```python
from build123d import *

# Parameters (mm, degrees)
SKETCH1_W           = 21
SKETCH1_H           = 15
BOSS_EXTRUDE1_DEPTH = 15
SKETCH3_W           = 18
SKETCH3_H           = 7
CUT_EXTRUDE1_DEPTH  = 3
SKETCH4_W           = 7
SKETCH4_H           = 7
BOSS_EXTRUDE3_DEPTH = 9
FILLET2_R           = 1


with BuildPart() as part:
    # Sketch1 → Boss-Extrude1 (new body)
    with BuildSketch(Plane(origin=(0, 0, 0), x_dir=(1, 0, 0), z_dir=(0, 1, 0))):
        Rectangle(SKETCH1_W, SKETCH1_H)
    extrude(amount=BOSS_EXTRUDE1_DEPTH)

    # Sketch3 → Cut-Extrude1 (cut)
    with BuildSketch(Plane(origin=(0, 15, 0), x_dir=(1, 0, 0), z_dir=(0, 1, 0))):
        Rectangle(SKETCH3_W, SKETCH3_H)
    extrude(amount=-CUT_EXTRUDE1_DEPTH, mode=Mode.SUBTRACT)

    # Sketch4 → Boss-Extrude3 (add)
    with BuildSketch(Plane(origin=(0, 12, 0), x_dir=(1, 0, 0), z_dir=(0, 1, 0))):
        with Locations((-5.5, 0)):
            Rectangle(SKETCH4_W, SKETCH4_H)
    extrude(amount=BOSS_EXTRUDE3_DEPTH)

    # Fillet2
    fillet2_edges = [part.edges().sort_by_distance(p)[0] for p in [
        (-9, 21, 0),
        (-5.5, 21, 3.5),
        (-2, 21, 0),
        (-5.5, 21, -3.5),
    ]]
    fillet(fillet2_edges, radius=FILLET2_R)


solid = part.part
```
Check sheet for the modelled part. Datum: model origin and axes. Units: mm. A direction names the side the tool comes from. Coordinates: 2 decimals unless noted, no trailing zeros. Loops run counter-clockwise (first coordinate to the right, second up) from the corner with the lowest first, then second, coordinate; pieces in that order, holes last.
1) Sectioned sample at C-C (y = 13.5). Record the boundary of the cut face in (x, z).
2) Sectioned sample at B-B (x = -7). Record the boundary of the cut face in (y, z).
3) Access from +Z, -Z, +X, -X, +Y, -Y to the whole of each face (thin tool, end or side, straight path). Record for faces 5 (the face through (-9, 17, 0)), 6 (the face through (-6, 17, -3.5)), 7 (the face through (3, 14, 3.5)), 8 (the face through (-6, 17, 3.5)).
4) Gauge pin test, flat ends, axial feed: pin 1 (1.5 mm diameter, centred on y = 17, z = 0, fed in from -X); pin 2 (2 mm diameter, centred on y = 16.5, z = 1.5, fed in from +X); pin 3 (4 mm diameter, centred on x = -4.5, y = 18.5, fed in from +Z). Record the tip position at first contact, or that the pin passes through.
5) Sectioned sample at D-D (y = 17). Record the boundary of the cut face in (x, z), and give its area (3 significant figures).
6) Sectioned sample at A-A (z = 1). Record the boundary of the cut face in (x, y), and give its area (3 significant figures).
7) Material ranges on probe 1 along Z at (x, y) = (4.5, 14.75); probe 2 along Y at (x, z) = (5, 3.25); probe 3 along Y at (x, z) = (-2.25, 6), recorded low to high.
8) Release check for a two-part mould opening along X. For faces 1 (the face through (0, 0, 0)), 2 (the face through (3, 12, 0)), 3 (the face through (10.5, 7, 0)), 4 (the face through (-2, 16, 0)) record: released by +X, released by -X, zero draft, split by the parting line, or undercut.
Check sheet entries:
1. outline: (-10.5, -7.5) - (10.5, -7.5) - (10.5, 7.5) - (-10.5, 7.5) - close; hole (-2, -3.5) - (9, -3.5) - (9, 3.5) - (-2, 3.5) - close
2. outline: (0, -7.5) - (15, -7.5) - (15, -3.5) - (20, -3.5) arc R1 ccw to (21, -2.5) - (21, 2.5) arc R1 ccw to (20, 3.5) - (15, 3.5) - (15, 7.5) - (0, 7.5) - close
3. face 5: +Z, -Z, -X, +Y
3. face 6: -Z, +X, -X, +Y
3. face 7: +Y
3. face 8: +Z, +X, -X, +Y
4. pin 1: stops at x = -9
4. pin 2: stops at x = -2
4. pin 3: stops at z = 3.5
5. outline: (-9, -3.5) - (-2, -3.5) - (-2, 3.5) - (-9, 3.5) - close
5. area: 49.0 mm2
6. outline: (-10.5, 0) - (10.5, 0) - (10.5, 15) - (9, 15) - (9, 12) - (-2, 12) - (-2, 20) arc R1 ccw to (-3, 21) - (-8, 21) arc R1 ccw to (-9, 20) - (-9, 15) - (-10.5, 15) - close
6. area: 324 mm2
7. probe 1: z = -7.5 to -3.5, 3.5 to 7.5
7. probe 2: y = 0 to 12
7. probe 3: y = 0 to 15
8. face 1: zero draft
8. face 2: undercut
8. face 3: released by +X
8. face 4: undercut
